The model under review builds one solid part; all positions refer to its coordinate system, in mm. Face numbers are marked on the shaded views. A direction names the side the tool comes from. Give positions to 0.01 mm unless a question says otherwise; leave off trailing zeros. Loops run counter-clockwise (first coordinate to the right, second up) from the corner with the lowest first, then second, coordinate; pieces in that order, holes last. Notation, with made-up numbers: (31, -38) - (36, -38) arc R36 cw to (36, 1) - close; hole circle Ø8 at (31, 66.5). An arc over 180 degrees is marked (long way). Return JSON: item names as keys, results as strings. Group by question number.
from build123d import *

# Parameters (mm, degrees)
BOSS_EXTRUDE1_DEPTH = 20
BOSS_EXTRUDE2_DEPTH = 31
SKETCH8_R           = 15
SKETCH8_R_2         = 11
CUT_EXTRUDE4_DEPTH  = 6
SKETCH8_2_R         = 11
CUT_EXTRUDE5_DEPTH  = 134.645052284
SKETCH10_R          = 6
SKETCH9_R           = 7
CUT_EXTRUDE6_DEPTH  = 134.645052321
SKETCH12_R          = 15
BOSS_EXTRUDE3_DEPTH = 1


with BuildPart() as part:
    # Sketch1 → Boss-Extrude1 (new body)
    with BuildSketch(Plane.XY):
        with BuildLine():
            Line((-50, 108.561575886), (-50, -23.561575886))
            ThreePointArc((-50, -23.561575886), (0, -35), (50, -23.561575886))
            Line((50, -23.561575886), (50, 108.561575886))
            ThreePointArc((50, 108.561575886), (0, 120), (-50, 108.561575886))
        make_face()
    extrude(amount=BOSS_EXTRUDE1_DEPTH)

    # Sketch2 → Boss-Extrude2 (add)
    with BuildSketch(Plane.XY.offset(20)):
        with BuildLine():
            Line((-50, 55), (-50, -23.561575886))
            ThreePointArc((-50, -23.561575886), (-41.631074926, -27.200063435), (-33, -30.163514831))
            Line((-33, -30.163514831), (-33, 55))
            Line((-33, 55), (-50, 55))
        make_face()
        with BuildLine():
            Line((33, 55), (33, -30.163514831))
            ThreePointArc((33, -30.163514831), (41.631074926, -27.200063435), (50, -23.561575886))
            Line((50, -23.561575886), (50, 55))
            Line((50, 55), (33, 55))
        make_face()
    extrude(amount=BOSS_EXTRUDE2_DEPTH)

    # Sketch8 → Cut-Extrude4 (cut)
    with BuildSketch(Plane.XY.offset(20)):
        Circle(SKETCH8_R)
        Circle(SKETCH8_R_2, mode=Mode.SUBTRACT)
    extrude(amount=-CUT_EXTRUDE4_DEPTH, mode=Mode.SUBTRACT)

    # Sketch8_2 → Cut-Extrude5 (cut, through all)
    with BuildSketch(Plane.XY.offset(20)):
        Circle(SKETCH8_2_R)
    extrude(amount=-CUT_EXTRUDE5_DEPTH, mode=Mode.SUBTRACT)

    # Sketch10 → Cut-Loft1 section 0
    with BuildSketch(Plane.ZY.offset(50)):
        with Locations((36, 41)):
            Circle(SKETCH10_R)
    # Sketch9 → Cut-Loft1 section 1
    with BuildSketch(Plane(origin=(50, 0, 0), x_dir=(0, 0, -1), z_dir=(1, 0, 0))):
        with Locations((-36, 41)):
            Circle(SKETCH9_R)
    loft(mode=Mode.SUBTRACT)

    # Sketch11 → Cut-Extrude6 (cut, through all)
    with BuildSketch(Plane.XY.offset(20)):
        with BuildLine():
            ThreePointArc((30.545454545, 91.010852136), (0, 96), (-30.545454545, 91.010852136))
            ThreePointArc((-30.545454545, 91.010852136), (-35.584237678, 80.881159913), (-25.454545455, 75.84237678))
            ThreePointArc((-25.454545455, 75.84237678), (0, 80), (25.454545455, 75.84237678))
            ThreePointArc((25.454545455, 75.84237678), (35.584237678, 80.881159913), (30.545454545, 91.010852136))
        make_face()
    extrude(amount=-CUT_EXTRUDE6_DEPTH, mode=Mode.SUBTRACT)

    # Sketch12 → Boss-Extrude3 (add)
    with BuildSketch(Plane.XY.offset(20)):
        with BuildLine():
            Line((-33, 55), (33, 55))
            Line((33, 55), (33, -30.163514831))
            ThreePointArc((33, -30.163514831), (0, -35), (-33, -30.163514831))
            Line((-33, -30.163514831), (-33, 55))
        make_face()
        Circle(SKETCH12_R, mode=Mode.SUBTRACT)
    extrude(amount=BOSS_EXTRUDE3_DEPTH)


solid = part.part
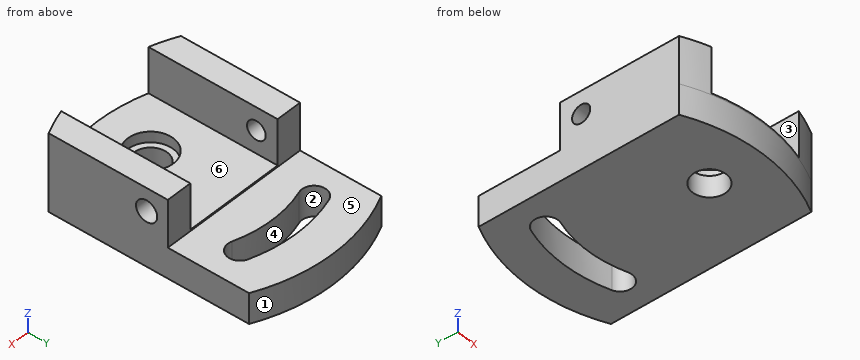
Item 1: Take a section at A-A (z = 4). State the section outline as (x, y) points, then the cut area to 3 significant figures.
Item 2: Take a section at D-D (y = 0). State the section outline as (x, z) points, then the cut area to 3 significant figures.
Item 3: For L1, parallel to X at y = 30, z = 47.5; L2, parallel to Z at x = 40, y = 99; L3, parallel to Z at x = -31, y = -22.5, list the stretches that pass through material, from the lowest coordinate up. Write a range as from..to.
Item 4: Tool access review of the marked faces 4, 5 and 6: name each direction out of +Z, -Z, +X, -X, +Y, -Y from which nothing blocks a thin tool from reaching the whole face with its end or side.
Item 5: Take a section at B-B (y = -21). State the section outline as (x, z) points, then the cut area to 3 significant figures.
Item 6: Take a section at C-C (x = 28.5). State the section outline as (y, z) points.
Item 7: Mouldability with a two-part tool opening along Y and no side actions: class the marked faces 1, 2 and 3 as +Y half, -Y half, draft (parallel to the pull), parting line (faces both ways), or undercut.
Item 8: For P1, Ø24, axis at x = 0, y = 0, coming from the +Z side; P2, Ø20, axis at x = -4.5, y = 24, coming from the +Z side; P3, Ø25, axis at x = -21, z = 30, coming from the +Y side, all flat-tipped, find the tip position at first contact; note any pin that passes through.
Check sheet entries:
{
 "1": {"outline": "(-50, -23.56) arc R115 ccw to (50, -23.56) - (50, 108.56) arc R115 ccw to (-50, 108.56) - close; hole (-30.55, 91.01) arc R8 ccw to (-25.45, 75.84) arc R80 cw to (25.45, 75.84) arc R8 ccw to (30.55, 91.01) arc R96 ccw to start; hole circle Ø22 at (0, 0)", "area": "13,300 mm^2"},
 "2": {"outline": "(-50, 0) - (-11, 0) - (-11, 14) - (-15, 14) - (-15, 21) - (-33, 21) - (-33, 51) - (-50, 51) - close; (11, 0) - (50, 0) - (50, 51) - (33, 51) - (33, 21) - (15, 21) - (15, 14) - (11, 14) - close", "area": "2,600 mm^2"},
 "3": {"L1": "x = -50..-33, 33..50", "L2": "z = 0..20", "L3": "z = 0..21"},
 "4": {"face 4": "+Z, -Z", "face 5": "+Z, +X, -X, +Y", "face 6": "+Z, +Y, -Y"},
 "5": {"outline": "(-50, 0) - (50, 0) - (50, 51) - (33, 51) - (33, 21) - (-33, 21) - (-33, 51) - (-50, 51) - close", "area": "3,120 mm^2"},
 "6": {"outline": "(-31.41, 0) - (75.44, 0) - (75.44, 20) - (55, 20) - (55, 21) - (-31.41, 21) - close; (91.67, 0) - (116.41, 0) - (116.41, 20) - (91.67, 20) - close"},
 "7": {"face 1": "+Y half", "face 2": "undercut", "face 3": "draft"},
 "8": {"P1": "stops at z = 14", "P2": "stops at z = 21", "P3": "stops at y = 119.2"}
}
